Can you work these out from the model? Positions are in its coordinate system, mm. A direction names the side the tool comes from. Give positions to 0.01 mm unless a question says otherwise; leave off trailing zeros. Write each loop counter-clockwise with the first axis right and the second up, starting at its lowest first coordinate (ties: lowest second). Pieces come first, ordered by that corner, then holes. Notation, with made-up numbers: M 88,35 L 133,35 A13 ccw 133,58 Z; hole C 88,18.25 d9. An arc over 180 degrees is marked long. Write each question's results on one line, items separated by ' | '.
from build123d import *

# Parameters (mm, degrees)
F0_W     = 558.8
F0_H     = 374.65
F0_W_2   = 38.1
F0_W_3   = 482.6
F0_H_2   = 19.05
F0_H_3   = 184.15
F0_H_4   = 12.7
F1_DEPTH = 38.1
F2_DEPTH = 914.4
F3_DEPTH = 914.4


with BuildPart() as f1:
    # F0 (on Top) → F1 (new body)
    with BuildSketch(Plane.XY):
        with Locations((558.8, 136.525)):
            Rectangle(F0_W, F0_H)
        with Locations((895.35, 136.525)):
            Rectangle(F0_W_2, F0_H)
        with Locations((-558.8, 136.525)):
            Rectangle(F0_W, F0_H)
        with Locations((-895.35, 136.525)):
            Rectangle(F0_W_2, F0_H)
        with Locations((0, 136.525)):
            Rectangle(F0_W_3, F0_H)
        with Locations((895.35, -60.325)):
            Rectangle(F0_W_2, F0_H_2)
        with Locations((-895.35, -60.325)):
            Rectangle(F0_W_2, F0_H_2)
        with Locations((260.35, 136.525)):
            Rectangle(F0_W_2, F0_H)
        with Locations((895.35, -161.925)):
            Rectangle(F0_W_2, F0_H_3)
        with Locations((-895.35, -263.525)):
            Rectangle(F0_W_2, F0_H_2)
        with Locations((857.25, 136.525)):
            Rectangle(F0_W_2, F0_H)
        Polygon((-914.4, -323.85), (914.4, -323.85), (914.4, -273.05), (876.3, -273.05), (876.3, -285.75), (838.2, -285.75), (838.2, -273.05), (279.4, -273.05), (279.4, -285.75), (241.3, -285.75), (241.3, -273.05), (-241.3, -273.05), (-241.3, -285.75), (-279.4, -285.75), (-279.4, -273.05), (-838.2, -273.05), (-838.2, -285.75), (-876.3, -285.75), (-876.3, -273.05), (-914.4, -273.05), align=None)
        with Locations((-895.35, -161.925)):
            Rectangle(F0_W_2, F0_H_3)
        with Locations((895.35, -263.525)):
            Rectangle(F0_W_2, F0_H_2)
        with Locations((-857.25, 136.525)):
            Rectangle(F0_W_2, F0_H)
        with Locations((-260.35, 136.525)):
            Rectangle(F0_W_2, F0_H)
        with Locations((-558.8, -60.325)):
            Rectangle(F0_W, F0_H_2)
        with Locations((-558.8, -161.925)):
            Rectangle(F0_W, F0_H_3)
        with Locations((-260.35, -161.925)):
            Rectangle(F0_W_2, F0_H_3)
        with Locations((0, -161.925)):
            Rectangle(F0_W_3, F0_H_3)
        with Locations((558.8, -161.925)):
            Rectangle(F0_W, F0_H_3)
        with Locations((260.35, -161.925)):
            Rectangle(F0_W_2, F0_H_3)
        with Locations((857.25, -161.925)):
            Rectangle(F0_W_2, F0_H_3)
        with Locations((558.8, -60.325)):
            Rectangle(F0_W, F0_H_2)
        with Locations((-857.25, -161.925)):
            Rectangle(F0_W_2, F0_H_3)
        with Locations((-857.25, -60.325)):
            Rectangle(F0_W_2, F0_H_2)
        with Locations((-857.25, -263.525)):
            Rectangle(F0_W_2, F0_H_2)
        with Locations((-857.25, -279.4)):
            Rectangle(F0_W_2, F0_H_4)
        with Locations((-558.8, -263.525)):
            Rectangle(F0_W, F0_H_2)
        with Locations((0, -60.325)):
            Rectangle(F0_W_3, F0_H_2)
        with Locations((0, -263.525)):
            Rectangle(F0_W_3, F0_H_2)
        with Locations((-260.35, -263.525)):
            Rectangle(F0_W_2, F0_H_2)
        with Locations((-260.35, -279.4)):
            Rectangle(F0_W_2, F0_H_4)
        with Locations((-260.35, -60.325)):
            Rectangle(F0_W_2, F0_H_2)
        with Locations((260.35, -60.325)):
            Rectangle(F0_W_2, F0_H_2)
        with Locations((260.35, -279.4)):
            Rectangle(F0_W_2, F0_H_4)
        with Locations((260.35, -263.525)):
            Rectangle(F0_W_2, F0_H_2)
        with Locations((558.8, -263.525)):
            Rectangle(F0_W, F0_H_2)
        with Locations((857.25, -60.325)):
            Rectangle(F0_W_2, F0_H_2)
        with Locations((857.25, -263.525)):
            Rectangle(F0_W_2, F0_H_2)
        with Locations((857.25, -279.4)):
            Rectangle(F0_W_2, F0_H_4)
    extrude(amount=F1_DEPTH)

    # F0 (on Top) → F2 (join)
    with BuildSketch(Plane.XY):
        with Locations((-260.35, -263.525)):
            Rectangle(F0_W_2, F0_H_2)
        with Locations((-260.35, -60.325)):
            Rectangle(F0_W_2, F0_H_2)
        with Locations((-260.35, -161.925)):
            Rectangle(F0_W_2, F0_H_3)
        with Locations((-260.35, -279.4)):
            Rectangle(F0_W_2, F0_H_4)
        with Locations((-260.35, 136.525)):
            Rectangle(F0_W_2, F0_H)
    extrude(amount=-F2_DEPTH)

    # F0 (on Top) → F3 (join)
    with BuildSketch(Plane.XY):
        with Locations((-857.25, -263.525)):
            Rectangle(F0_W_2, F0_H_2)
        with Locations((-857.25, 136.525)):
            Rectangle(F0_W_2, F0_H)
        with Locations((-857.25, -60.325)):
            Rectangle(F0_W_2, F0_H_2)
        with Locations((-857.25, -279.4)):
            Rectangle(F0_W_2, F0_H_4)
        with Locations((-857.25, -161.925)):
            Rectangle(F0_W_2, F0_H_3)
    extrude(amount=-F3_DEPTH)


solid = f1.part
Item 1: For faces 1 (the face through (-241.3, 15, -451)), 2 (the face through (-858, -285.75, -451)), 3 (the face through (-13, -323.85, 19)), which set-ups out of +Z, -Z, +X, -X, +Y, -Y let a thin tool reach every point of the face, with its end or its side?
Geometry says:
face 1: -Z, +X, +Y, -Y | face 2: -Z, +X, -X, -Y | face 3: +Z, -Z, +X, -X, -Y
Item 2: If I drill on line 1 (X direction, y = -8.5, z = -463); line 2 (Z direction, x = -208, y = -84.5), over which ranges is the centre line in solid material (lowest first)? Write a range as from..to.
Geometry says:
line 1: x = -876.3..-838.2, -279.4..-241.3 | line 2: z = 0..38.1
Item 3: I want a section at B-B, the plane y = -19.5. Please give me the cut outline in (x, z), and give its area (3 significant figures).
Geometry says:
outline: M -914.4,0 L -876.3,0 L -876.3,-914.4 L -838.2,-914.4 L -838.2,0 L -279.4,0 L -279.4,-914.4 L -241.3,-914.4 L -241.3,0 L 914.4,0 L 914.4,38.1 L -914.4,38.1 Z | area: 139,000 mm2
Item 4: I want a section at A-A, the plane z = -264. Please give me the cut outline in (x, y).
Geometry says:
outline: M -876.3,-285.75 L -838.2,-285.75 L -838.2,323.85 L -876.3,323.85 Z; M -279.4,-285.75 L -241.3,-285.75 L -241.3,323.85 L -279.4,323.85 Z
Item 5: I want a section at C-C, the plane x = 354.5. Please give me the cut outline in (y, z), and give its area (3 significant figures).
Geometry says:
outline: M -323.85,0 L 323.85,0 L 323.85,38.1 L -323.85,38.1 Z | area: 24,700 mm2
Item 6: Thinking about a two-plate mould opening in X: for faces 4 (the face through (-876.3, 23, -451)), 5 (the face through (-261, -285.75, -451)), 6 (the face through (-279.4, 23, -451)), 7 (the face through (-838.2, 15, -451)), which applies, +X half, -X half, draft (parallel to the pull), parting line (faces both ways), or undercut?
Geometry says:
face 4: -X half | face 5: draft | face 6: undercut | face 7: undercut
Item 7: I'm going to push flat-ended pins straight in: pin 1 (19 mm diameter, centred on x = -256, z = -418, fed in from -Y); pin 2 (2 mm diameter, centred on y = -109, z = -440, fed in from -X); pin 3 (12 mm diameter, centred on x = -373.5, y = 179.5, fed in from -Z). Where does each tip first touch, or does it pass through?
Geometry says:
pin 1: stops at y = -285.75 | pin 2: stops at x = -876.3 | pin 3: stops at z = 0
